from build123d import *

# Parameters (mm, degrees)
PAD_DEPTH       = 3
PAD001_DEPTH    = 5
SKETCH002_R     = 1.6
POCKET_DEPTH    = 110.001
SKETCH003_R     = 3
SKETCH003_R_2   = 1.5
PAD002_DEPTH    = 5
CHAMFER_SIZE    = 3
CHAMFER001_SIZE = 2


with BuildPart() as part:
    # Sketch → Pad (new body)
    with BuildSketch(Plane.XY):
        Polygon((0, 0), (200, 0), (200, 15), (137.5, 60), (137.5, 110), (62.5, 110), (62.5, 60), (0, 15), align=None)
    extrude(amount=PAD_DEPTH)

    # Sketch001 (on Face1 of Pad) → Pad001 (join)
    with BuildSketch(Plane.XZ):
        Polygon((0, 3), (0, 20), (10, 20), (10, 7.5), (190, 7.5), (190, 20), (200, 20), (200, 3), align=None)
    extrude(amount=-PAD001_DEPTH)

    # Sketch002 (on Face14 of Pad001) → Pocket (cut, through all)
    with BuildSketch(Plane.XZ):
        with Locations((7.5, 7.5)):
            Circle(SKETCH002_R)
        with Locations((192.5, 7.5)):
            Circle(SKETCH002_R)
    extrude(amount=-POCKET_DEPTH, mode=Mode.SUBTRACT)

    # Sketch003 (on Face7 of Pocket) → Pad002 (join)
    with BuildSketch(Plane.XY.offset(3)):
        with Locations((76.5, 99.5)):
            Circle(SKETCH003_R)
        with Locations((76.5, 99.5)):
            Circle(SKETCH003_R_2, mode=Mode.SUBTRACT)
        with Locations((123.5, 99.5)):
            Circle(SKETCH003_R)
        with Locations((123.5, 99.5)):
            Circle(SKETCH003_R_2, mode=Mode.SUBTRACT)
        with Locations((123.5, 35)):
            Circle(SKETCH003_R)
        with Locations((123.5, 35)):
            Circle(SKETCH003_R_2, mode=Mode.SUBTRACT)
        with Locations((76.5, 35)):
            Circle(SKETCH003_R)
        with Locations((76.5, 35)):
            Circle(SKETCH003_R_2, mode=Mode.SUBTRACT)
    extrude(amount=PAD002_DEPTH)

    # Chamfer
    chamfer_edges = [part.edges().sort_by_distance(p)[0] for p in [
        (10, 2.5, 7.5),
        (190, 2.5, 7.5),
        (190, 2.5, 20),
        (10, 2.5, 20),
    ]]
    chamfer(chamfer_edges, length=CHAMFER_SIZE)

    # Chamfer001
    chamfer001_edges = [part.edges().sort_by_distance(p)[0] for p in [
        (100, 5, 3),
    ]]
    chamfer(chamfer001_edges, length=CHAMFER001_SIZE)


solid = part.part
Verification items for the finished model (mm, model axes). A direction names the side the tool comes from. Coordinates: 2 decimals unless noted, no trailing zeros. Write each loop counter-clockwise with the first axis right and the second up, starting at its lowest first coordinate (ties: lowest second). Pieces come first, ordered by that corner, then holes. Notation, with made-up numbers: M 74,-33 L 118,-33 A19 cw 118,-15 Z; hole C 15,-15 d7. An arc over 180 degrees is marked long. Use a Markdown table: item, result.
Q1. Sectioned sample at A-A, the plane x = 28. Record the boundary of the cut face in (y, z), plus the area to 3 significant figures.
Reply:
| item | result |
|---|---|
| outline | M 0,0 L 35.16,0 L 35.16,3 L 7,3 L 5,5 L 5,7.5 L 0,7.5 Z |
| area | 130 mm² |
Q2. Sectioned sample at C-C, the plane x = 55.5. Record the boundary of the cut face in (y, z).
Reply:
| item | result |
|---|---|
| outline | M 0,0 L 54.96,0 L 54.96,3 L 7,3 L 5,5 L 5,7.5 L 0,7.5 Z |
Q3. Set-up check for faces 5 (the face through (75.85, 96.57, 5.46)), 6 (the face through (190, 2, 14)), 7 (the face through (196, 2, 20)): record each of +Z, -Z, +X, -X, +Y, -Y from which the full face is reachable in a straight line by a thin tool's end or side.
Reply:
| item | result |
|---|---|
| face 5 | +Z |
| face 6 | +Z, +Y, -Y |
| face 7 | +Z, +X, -X, +Y, -Y |
Q4. Sectioned sample at B-B, the plane y = 46.5. Record the boundary of the cut face in (x, z), plus the area to 4 significant figures.
Reply:
| item | result |
|---|---|
| outline | M 43.75,0 L 156.25,0 L 156.25,3 L 43.75,3 Z |
| area | 337.5 mm² |
Q5. Sectioned sample at D-D, the plane y = 92. Record the boundary of the cut face in (x, z), plus the area to 3 significant figures.
Reply:
| item | result |
|---|---|
| outline | M 62.5,0 L 137.5,0 L 137.5,3 L 62.5,3 Z |
| area | 225 mm² |
Q6. Thickness scan on line 1 (Y direction, x = 76.5, z = 5.4); line 2 (Z direction, x = 124.5, y = 99); line 3 (Y direction, x = 76.5, z = 4.05). Record the ranges inside material, lowest first.
Reply:
| item | result |
|---|---|
| line 1 | y = 0 to 5, 32 to 33.5, 36.5 to 38, 96.5 to 98, 101 to 102.5 |
| line 2 | z = 0 to 3 |
| line 3 | y = 0 to 5.95, 32 to 33.5, 36.5 to 38, 96.5 to 98, 101 to 102.5 |
Q7. Draft check along Y on faces 1 (the face through (74.29, 37.03, 5.46)), 2 (the face through (125, 98, 8)), 3 (the face through (126.36, 35.9, 5.46)), 4 (the face through (169.188, 37.185, 1.479)). Enter one of: +Y half, -Y half, draft (parallel to the pull), parting line (faces both ways), or undercut.
Reply:
| item | result |
|---|---|
| face 1 | undercut |
| face 2 | draft |
| face 3 | undercut |
| face 4 | +Y half |
Q8. Go/stop test with flat-tipped pins: P1, Ø2.5, axis at x = 76.5, y = 99.5, coming from the +Z side; P2, Ø5, axis at x = 124, y = 33.5, coming from the +Z side; P3, Ø7.5, axis at x = 126.5, z = 13, coming from the +Y side; P4, Ø1.5, axis at x = 134, y = 2.5, coming from the +Z side. Record where each tip stops, or that it passes through.
Reply:
| item | result |
|---|---|
| P1 | stops at z = 3 |
| P2 | stops at z = 8 |
| P3 | passes through |
| P4 | stops at z = 7.5 |
